```python
from build123d import *

# Parameters (mm, degrees)
FILLET1_R = 1
FILLET2_R = 10


with BuildPart() as part:
    # Sketch1 → Revolve1 (revolve)
    with BuildSketch(Plane.XY, mode=Mode.PRIVATE) as revolve1_sk:
        Polygon((0, 0), (0, 10), (32, 10), (32, 20), (52, 10), (72, 20), (72, 10), (104, 10), (104, 0), align=None)
    revolve(revolve1_sk.sketch.rotate(Axis((0, 0, 0), (1, 0, 0)), 90), axis=Axis((0, 0, 0), (1, 0, 0)))

    # Fillet1
    fillet1_edges = [part.edges().sort_by_distance(p)[0] for p in [
        (32, 0, -10),
        (72, 0, -10),
    ]]
    fillet(fillet1_edges, radius=FILLET1_R)

    # Fillet2
    fillet2_edges = [part.edges().sort_by_distance(p)[0] for p in [
        (52, 0, -10),
    ]]
    fillet(fillet2_edges, radius=FILLET2_R)


solid = part.part
```
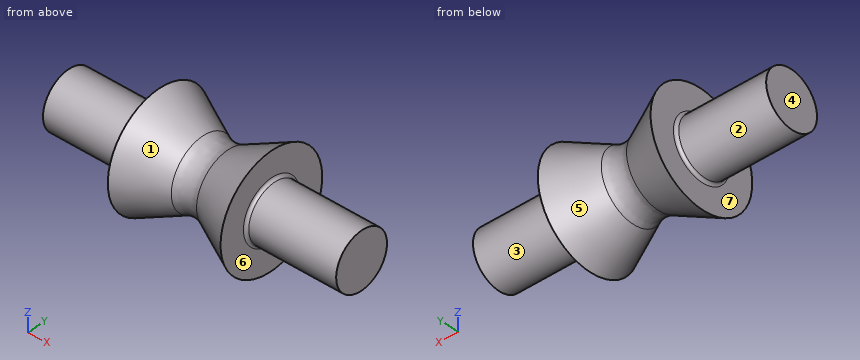
Build history of the part. All positions in model axes, mm. Face numbers are marked on the shaded views. A direction names the side the tool comes from. Coordinates: 2 decimals unless noted, no trailing zeros.
Item 1: Mould opens along X. For the marked faces 5, 6 and 7 say: released by +X, released by -X, zero draft, split by the parting line, or undercut.
Filled in:
face 5: undercut
face 6: released by +X
face 7: released by -X
Item 2: Drop flat-ended pins along their axis: pin 1 Ø3 at (y, z) = (-6.5, 10.5) entering from +X; pin 2 Ø12 at (x, y) = (56, 7) entering from +Z; pin 3 Ø1 at (x, z) = (14.5, 4) entering from -Y. Give the stop position or say it passes through.
Filled in:
pin 1: stops at x = 72.01
pin 2: stops at z = 14.04
pin 3: stops at y = -9.37
Item 3: Drill centre lines: L1, parallel to X at y = -3, z = -14.5; L2, parallel to X at y = -16.5, z = -8.5; L3, parallel to Z at x = 76, y = 2. Where is each one in solid material? Low to high.
Filled in:
L1: x = 32 to 42.39, 61.61 to 72
L2: x = 32 to 34.88, 69.12 to 72
L3: z = -9.8 to 9.8
Item 4: Tool access for the marked faces 1, 2, 3 and 4: list every direction of +Z, -Z, +X, -X, +Y, -Y with a clear straight run to the whole face (end or side of a thin tool).
Filled in:
face 1: none
face 2: -X
face 3: +X
face 4: +Z, -Z, -X, +Y, -Y
